from build123d import *

# Parameters (mm, degrees)
SKETCH_1_W          = 20
SKETCH_1_H          = 20
SKETCH_1_W_2        = 17
SKETCH_1_H_2        = 17
EXTRUDE_1_DEPTH     = 110
SKETCH_2_R          = 2.7
CUT_EXTRUDE_1_DEPTH = 25
SKETCH_3_R          = 2.25
CUT_EXTRUDE_2_DEPTH = 20
SKETCH_5_R          = 5
CUT_EXTRUDE_4_DEPTH = 10
SKETCH_6_R          = 5
CUT_EXTRUDE_5_DEPTH = 10


with BuildPart() as part:
    # ｽｹｯﾁ1 → ﾎﾞｽ - 押し出し1 (new body)
    with BuildSketch(Plane.XY):
        Rectangle(SKETCH_1_W, SKETCH_1_H)
        Rectangle(SKETCH_1_W_2, SKETCH_1_H_2, mode=Mode.SUBTRACT)
    extrude(amount=EXTRUDE_1_DEPTH)

    # ｽｹｯﾁ2 → ｶｯﾄ - 押し出し1 (cut)
    with BuildSketch(Plane(origin=(10, 0, 0), x_dir=(0, 0, -1), z_dir=(1, 0, 0))):
        with Locations((-60, 0)):
            Circle(SKETCH_2_R)
        with Locations((-10, 0)):
            Circle(SKETCH_2_R)
    extrude(amount=-CUT_EXTRUDE_1_DEPTH, mode=Mode.SUBTRACT)

    # ｽｹｯﾁ3 → ｶｯﾄ - 押し出し2 (cut)
    with BuildSketch(Plane(origin=(0, 10, 0), x_dir=(1, 0, 0), z_dir=(0, 1, 0))):
        with Locations((0, -100)):
            Circle(SKETCH_3_R)
        with Locations((0, -80)):
            Circle(SKETCH_3_R)
        with Locations((0, -20)):
            Circle(SKETCH_3_R)
    extrude(amount=-CUT_EXTRUDE_2_DEPTH, mode=Mode.SUBTRACT)

    # ｽｹｯﾁ5 → ｶｯﾄ - 押し出し4 (cut)
    with BuildSketch(Plane(origin=(0, -10, 0), x_dir=(-1, 0, 0), z_dir=(0, -1, 0))):
        with Locations((0, -20)):
            Circle(SKETCH_5_R)
    extrude(amount=-CUT_EXTRUDE_4_DEPTH, mode=Mode.SUBTRACT)

    # ｽｹｯﾁ6 → ｶｯﾄ - 押し出し5 (cut)
    with BuildSketch(Plane.ZY.offset(10)):
        with Locations((10, 0)):
            Circle(SKETCH_6_R)
        with Locations((60, 0)):
            Circle(SKETCH_6_R)
    extrude(amount=-CUT_EXTRUDE_5_DEPTH, mode=Mode.SUBTRACT)


solid = part.part
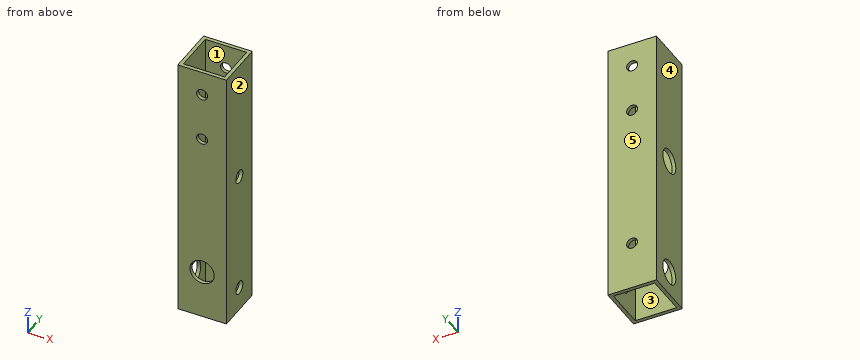
Could you check a few things on this model? Use its own coordinates, in mm. Face numbers are marked on the shaded views. A direction names the side the tool comes from. Give positions to 0.01 mm unless a question says otherwise; leave off trailing zeros. Loops run counter-clockwise (first coordinate to the right, second up) from the corner with the lowest first, then second, coordinate; pieces in that order, holes last. Notation, with made-up numbers: M 55,15 L 78,15 A16 cw 78,42 Z; hole C 8,21 d10. An arc over 180 degrees is marked long. Answer as a JSON object with one key per item and string values.
Q1. For P1, Ø6, axis at y = 0, z = 60, coming from the -X side, with a flat end and sliding along its axis, tell me the tip position at first contact or that it passes through.
Values found:
{"P1": "stops at x = 8.5"}
Q2. For the marked faces 1 and 2, which set-ups out of +Z, -Z, +X, -X, +Y, -Y let a thin tool reach every point of the face, with its end or its side?
Values found:
{"face 1": "+Z, -Z", "face 2": "+Z, -Z, +X, +Y, -Y"}
Q3. Suppose I cut it at C-C, the plane x = 0. State how many separate pieces and enclosed holes the cut face has, plus the area to 3 significant figures.
Values found:
{"separate pieces": "8", "enclosed holes": "0", "area": "281 mm²"}
Q4. If I drill on probe 1 along Z at (x, y) = (0, -9.7); probe 2 along Z at (x, y) = (0, 9.75); probe 3 along Y at (x, z) = (-8.95, 10), over which ranges is the centre line in solid material (lowest first)? Write a range as [from, to].
Values found:
{"probe 1": "z = [0, 15], [25, 77.75], [82.25, 97.75], [102.25, 110]", "probe 2": "z = [0, 17.75], [22.25, 77.75], [82.25, 97.75], [102.25, 110]", "probe 3": "y = [-10, -5], [5, 10]"}
Q5. Suppose I cut it at D-D, the plane y = 0. List the corners of the cut face in (x, z) for me.
Values found:
{"outline": "M -10,0 L -8.5,0 L -8.5,5 L -10,5 Z; M -10,15 L -8.5,15 L -8.5,55 L -10,55 Z; M -10,65 L -8.5,65 L -8.5,110 L -10,110 Z; M 8.5,0 L 10,0 L 10,7.3 L 8.5,7.3 Z; M 8.5,12.7 L 10,12.7 L 10,57.3 L 8.5,57.3 Z; M 8.5,62.7 L 10,62.7 L 10,110 L 8.5,110 Z"}
Q6. Suppose I cut it at A-A, the plane y = -7. List the corners of the cut face in (x, z) for me, plus the area to 3 significant figures.
Values found:
{"outline": "M -10,0 L -8.5,0 L -8.5,110 L -10,110 Z; M 8.5,0 L 10,0 L 10,110 L 8.5,110 Z", "area": "330 mm²"}
Q7. If we mould it in two halves opening along X, with no side actions, what happens to the marked faces 3, 4 and 5? For each: pulls with the +X half, pulls with the -X half, needs draft (parallel to the pull), parting line crosses it, or undercut.
Values found:
{"face 3": "undercut", "face 4": "pulls with the -X half", "face 5": "needs draft"}
Q8. Suppose I cut it at B-B, the plane z = 100. List the corners of the cut face in (x, y) for me, plus the area to 3 significant figures.
Values found:
{"outline": "M -10,-10 L -2.25,-10 L -2.25,-8.5 L -8.5,-8.5 L -8.5,8.5 L -2.25,8.5 L -2.25,10 L -10,10 Z; M 2.25,-10 L 10,-10 L 10,10 L 2.25,10 L 2.25,8.5 L 8.5,8.5 L 8.5,-8.5 L 2.25,-8.5 Z", "area": "97.5 mm²"}
